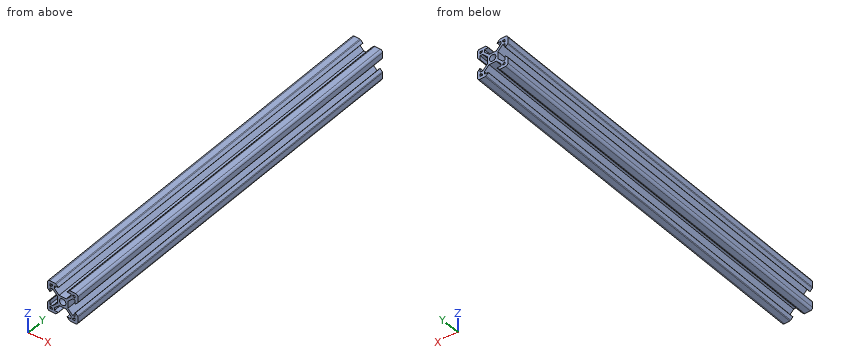
```python
from build123d import *

# Parameters (mm, degrees)
F0_R     = 2.1
F1_DEPTH = 254


with BuildPart() as f1:
    # F0 (on Front) → F1 (new body)
    with BuildSketch(Plane.XZ):
        with BuildLine():
            Line((-123.038144, 8.423504), (-126.198804, 11.584164))
            Line((-126.198804, 11.584164), (-126.198804, 16.262844))
            Line((-126.198804, 16.262844), (-123.038144, 19.423504))
            Line((-123.038144, 19.423504), (-121.398804, 19.423504))
            Line((-121.398804, 19.423504), (-121.398804, 16.813504))
            Line((-121.398804, 16.813504), (-121.288804, 16.813504))
            Line((-121.288804, 16.813504), (-119.83019, 18.272118))
            ThreePointArc((-119.83019, 18.272118), (-119.65894, 18.528413), (-119.598804, 18.830732))
            Line((-119.598804, 18.830732), (-119.598804, 22.423504))
            ThreePointArc((-119.598804, 22.423504), (-120.038144, 23.484164), (-121.098804, 23.923504))
            Line((-121.098804, 23.923504), (-124.691576, 23.923504))
            ThreePointArc((-124.691576, 23.923504), (-124.993896, 23.863369), (-125.25019, 23.692118))
            Line((-125.25019, 23.692118), (-126.708804, 22.233504))
            Line((-126.708804, 22.233504), (-126.708804, 22.123504))
            Line((-126.708804, 22.123504), (-124.098804, 22.123504))
            Line((-124.098804, 22.123504), (-124.098804, 20.484164))
            Line((-124.098804, 20.484164), (-127.259465, 17.323504))
            Line((-127.259465, 17.323504), (-131.938144, 17.323504))
            Line((-131.938144, 17.323504), (-135.098804, 20.484164))
            Line((-135.098804, 20.484164), (-135.098804, 22.123504))
            Line((-135.098804, 22.123504), (-132.488804, 22.123504))
            Line((-132.488804, 22.123504), (-132.488804, 22.233504))
            Line((-132.488804, 22.233504), (-133.947419, 23.692118))
            ThreePointArc((-133.947419, 23.692118), (-134.203713, 23.863369), (-134.506033, 23.923504))
            Line((-134.506033, 23.923504), (-138.098804, 23.923504))
            ThreePointArc((-138.098804, 23.923504), (-139.159465, 23.484164), (-139.598804, 22.423504))
            Line((-139.598804, 22.423504), (-139.598804, 18.830732))
            ThreePointArc((-139.598804, 18.830732), (-139.538669, 18.528413), (-139.367419, 18.272118))
            Line((-139.367419, 18.272118), (-137.908804, 16.813504))
            Line((-137.908804, 16.813504), (-137.798804, 16.813504))
            Line((-137.798804, 16.813504), (-137.798804, 19.423504))
            Line((-137.798804, 19.423504), (-136.159465, 19.423504))
            Line((-136.159465, 19.423504), (-132.998804, 16.262844))
            Line((-132.998804, 16.262844), (-132.998804, 11.584164))
            Line((-132.998804, 11.584164), (-136.159465, 8.423504))
            Line((-136.159465, 8.423504), (-137.798804, 8.423504))
            Line((-137.798804, 8.423504), (-137.798804, 11.033504))
            Line((-137.798804, 11.033504), (-137.908804, 11.033504))
            Line((-137.908804, 11.033504), (-139.367419, 9.574889))
            ThreePointArc((-139.367419, 9.574889), (-139.538669, 9.318595), (-139.598804, 9.016275))
            Line((-139.598804, 9.016275), (-139.598804, 5.423504))
            ThreePointArc((-139.598804, 5.423504), (-139.159465, 4.362844), (-138.098804, 3.923504))
            Line((-138.098804, 3.923504), (-134.506033, 3.923504))
            ThreePointArc((-134.506033, 3.923504), (-134.203713, 3.983639), (-133.947419, 4.154889))
            Line((-133.947419, 4.154889), (-132.488804, 5.613504))
            Line((-132.488804, 5.613504), (-132.488804, 5.723504))
            Line((-132.488804, 5.723504), (-135.098804, 5.723504))
            Line((-135.098804, 5.723504), (-135.098804, 7.362844))
            Line((-135.098804, 7.362844), (-131.938144, 10.523504))
            Line((-131.938144, 10.523504), (-127.259465, 10.523504))
            Line((-127.259465, 10.523504), (-124.098804, 7.362844))
            Line((-124.098804, 7.362844), (-124.098804, 5.723504))
            Line((-124.098804, 5.723504), (-126.708804, 5.723504))
            Line((-126.708804, 5.723504), (-126.708804, 5.613504))
            Line((-126.708804, 5.613504), (-125.25019, 4.154889))
            ThreePointArc((-125.25019, 4.154889), (-124.993896, 3.983639), (-124.691576, 3.923504))
            Line((-124.691576, 3.923504), (-121.098804, 3.923504))
            ThreePointArc((-121.098804, 3.923504), (-120.038144, 4.362844), (-119.598804, 5.423504))
            Line((-119.598804, 5.423504), (-119.598804, 9.016275))
            ThreePointArc((-119.598804, 9.016275), (-119.65894, 9.318595), (-119.83019, 9.574889))
            Line((-119.83019, 9.574889), (-121.288804, 11.033504))
            Line((-121.288804, 11.033504), (-121.398804, 11.033504))
            Line((-121.398804, 11.033504), (-121.398804, 8.423504))
            Line((-121.398804, 8.423504), (-123.038144, 8.423504))
        make_face()
        Polygon((-137.798804, 7.353504), (-137.258804, 7.353504), (-136.168804, 6.263504), (-136.168804, 5.723504), (-137.798804, 5.723504), align=None, mode=Mode.SUBTRACT)
        Polygon((-121.938804, 7.353504), (-121.398804, 7.353504), (-121.398804, 5.723504), (-123.028804, 5.723504), (-123.028804, 6.263504), align=None, mode=Mode.SUBTRACT)
        with Locations((-129.598804, 13.923504)):
            Circle(F0_R, mode=Mode.SUBTRACT)
        Polygon((-136.168804, 22.123504), (-136.168804, 21.583504), (-137.258804, 20.493504), (-137.798804, 20.493504), (-137.798804, 22.123504), align=None, mode=Mode.SUBTRACT)
        Polygon((-123.028804, 21.583504), (-123.028804, 22.123504), (-121.398804, 22.123504), (-121.398804, 20.493504), (-121.938804, 20.493504), align=None, mode=Mode.SUBTRACT)
    extrude(amount=F1_DEPTH)


solid = f1.part
```
Input: part model. Units: mm. Frame: model coordinates. Give positions to 0.01 mm unless a question says otherwise; leave off trailing zeros. Write item = value, one per line. Start each with the question number.
1. First-contact query: pin 1 Ø4 at (x, y) = (-131, -221.5) entering from -Z; pin 2 Ø3.5 at (x, y) = (-130.5, -96.5) entering from -Z; pin 3 Ø1 at (x, y) = (-133.5, -59) entering from +Z. Flat tips, straight axial feed; report the tip coordinate or a pass-through.
2. Section query A-A, the plane y = -83. Count the separate pieces of the cut face and the enclosed holes in it, then the cut area to 3 significant figures.
3. Ray query, L1, parallel to Z at x = -121.75, y = -29.5; L2, parallel to X at y = -109, z = 9.5; L3, parallel to Z at x = -125, y = -71. Return the intervals inside material, ascending.
Check sheet entries:
q1.pin_1 = 5.1
q1.pin_2 = 10.21
q1.pin_3 = 23.74
q2.separate_pieces = 1
q2.enclosed_holes = 5
q2.area = 152 mm2
q3.L1 = 3.92 to 5.72, 7.35 to 8.42, 19.42 to 20.49, 22.12 to 23.92
q3.L2 = -139.43 to -137.8, -135.08 to -132.96, -126.24 to -124.11, -121.4 to -119.76
q3.L3 = 3.99 to 5.72, 8.26 to 10.39, 17.46 to 19.58, 22.12 to 23.86
